Check sheet for the modelled part. Datum: model origin and axes. Units: mm. A direction names the side the tool comes from. Round coordinates to 2 decimals unless told otherwise and drop trailing zeros. Loops run counter-clockwise (first coordinate to the right, second up) from the corner with the lowest first, then second, coordinate; pieces in that order, holes last. Notation, with made-up numbers: (87.25, 67.5) - (107.25, 67.5) arc R19 cw to (107.25, 98.5) - close; hole circle Ø3 at (62.5, 38.25). An arc over 180 degrees is marked (long way). Answer in a Markdown table with one row per item. Add a question column.
(1) Access from +Z, -Z, +X, -X, +Y, -Y to the whole of each face (thin tool, end or side, straight path). Record for faces 5 (the flat face through (-39, 18, -33.975)), 6 (the flat face through (-39, 5.2, -51)), 7 (the flat face through (-39, 3, -56)).
(2) Cross-section at D-D on y = 11.5. Enter the section's corners in (x, z), then the cut area to 3 significant figures.
(3) Cross-section at B-B on z = -6. Enter the section's corners in (x, y).
(4) Cross-section at A-A on x = -43. Enter the section's corners in (y, z), then the cut area to 3 significant figures.
(5) Cross-section at C-C on x = -37.25. Enter the section's corners in (y, z).
(6) Gauge pin test, flat ends, axial feed: pin 1 (5 mm diameter, centred on x = -43, z = -50, fed in from +Y); pin 2 (12 mm diameter, centred on x = -33.5, z = -19.5, fed in from +Y); pin 3 (3 mm diameter, centred on x = -45, y = 19.5, fed in from +Z). Record the tip position at first contact, or that the pin passes through.
(7) Mould release check, pull along X, two halves, no side actions. Record for faces 1 (the cylindrical face through (-42.26, 2.64, -48.58)), 2 (the flat face through (-39, 21.2, -35)), 3 (the cylindrical face through (-43.35, 2.64, -4.44)), 4 (the cylindrical face through (-26.57, 2.64, -55.4)): +X half, -X half, draft (parallel to the pull), parting line (faces both ways), or undercut.
(8) Thickness scan on line 1 along Z through (x, y) = (-43, 3.05); line 2 along X through (y, z) = (1.5, -6); line 3 along Y through (x, z) = (-47, -17.5). Record the ranges inside material, lowest first.
Autodesk Inventor part; units mm, degrees
ref_plane "YZ Plane" through (0, 0, 0) normal (1, 0, 0) x (0, 1, 0)
ref_plane "XZ Plane" through (0, 0, 0) normal (0, 1, 0) x (-1, 0, 0)
ref_plane "XY Plane" through (0, 0, 0) normal (0, 0, 1) x (1, 0, 0)
sketch "Эскиз1" plane through (0, 0, 0) normal (0, 1, 0) x (-1, 0, 0)
  line L0 (0, 0) -> (52, 0)
  line L1 (52, 0) -> (52, -56)
  line L2 (52, -56) -> (0, -56)
  line L3 (0, -56) -> (0, 0)
  dimension "d0" = 56
  dimension "d9" = 52
extrude "Выдавливание1" add sketch "Эскиз1" along normal blind 5.2
ref_plane "РабПлоскость2" through (0, 3.2, -12) normal (0, -1, 0) x (1, 0, 0)
fillet "Сопряжение1" radius 2 4 edges at (0, 2.6, 0) (0, 2.6, -56) (-52, 2.6, -56) (-52, 2.6, 0)
ref_plane "РабПлоскость1" through (0, 0, -12) normal (1, 0, 0) x (0, 0, -1)
sketch "Эскиз4" plane through (0, 0, -12) normal (1, 0, 0) x (0, 0, -1)
  line L0 (34.9749, 5.2) -> (21.9749, 5.2)
  line L1 (21.9749, 21.2) -> (21.9749, 5.2)
  arc A0 (24.5222, 21.2) -> (34.9749, 5.2) centre (138.2876, 84.1082) ccw
  line L2 (21.9749, 21.2) -> (24.5222, 21.2)
  line L3 (44, 0) -> (44, 5.2)
  point P0 (-12, 0)
  dimension "d26" = 13
  dimension "d35" = 130
  dimension "d43" = 9.0251
extrude "Выдавливание4" add sketch "Эскиз4" against normal up to surface (52 mm away)
sketch "Эскиз5" plane through (0, 0, 0) normal (0, -1, 0) x (1, 0, 0)
  line L0 (0, 0) -> (-26, 0)
  line L1 (-26, 0) -> (-26, -56)
  line L2 (-26, -56) -> (0, -56)
  line L3 (0, -56) -> (0, 0)
  dimension "d37" = 26
extrude "Выдавливание5" cut sketch "Эскиз5" against normal blind 34
fillet "Сопряжение4" radius 2 2 edges at (-26, 2.6, 0) (-26, 2.6, -56)
fillet "Сопряжение5" radius 10 1 edges at (-39, 5.2, -33.9749)
sketch "Эскиз6" plane through (0, 5.2, 0) normal (0, 1, 0) x (1, 0, 0)
  circle A0 centre (-43, 6) radius 1.6
  circle A1 centre (-43, 50) radius 1.6
  line L0 (-52, 54) -> (-52, 46.9749)
  line L1 (-52, 23.9749) -> (-52, 2)
  line L2 (-50, 0) -> (-28, 0)
  line L3 (-28, 56) -> (-50, 56)
  point P0 (0, 0)
  dimension "d45" = 3.2
  dimension "d46" = 3.2
  dimension "d47" = 9
  dimension "d48" = 9
  dimension "d49" = 6
  dimension "d50" = 6
extrude "Выдавливание6" cut sketch "Эскиз6" against normal blind 40
properties part number "порожек"
Answers:
| question | item | result |
|---|---|---|
| 1 | face 5 | +Z, +X, -X, +Y |
| 1 | face 6 | -Z, +X, -X, +Y |
| 1 | face 7 | -Z, +X, -X, +Y, -Y |
| 2 | outline | (-52, -42.45) - (-26, -42.45) - (-26, -33.27) - (-52, -33.27) - close |
| 2 | area | 239 mm^2 |
| 3 | outline | (-52, 0) - (-44.6, 0) - (-44.6, 5.2) - (-52, 5.2) - close; (-41.4, 0) - (-26, 0) - (-26, 5.2) - (-41.4, 5.2) - close |
| 4 | outline | (0, -56) - (5.2, -56) - (5.2, -51.6) - (0, -51.6) - close; (0, -48.4) - (5.2, -48.4) - (5.2, -46.97) arc R130.01 cw to (21.2, -36.52) - (21.2, -33.97) - (15.2, -33.97) arc R10 cw to (5.2, -23.97) - (5.2, -7.6) - (0, -7.6) - close; (0, -4.4) - (5.2, -4.4) - (5.2, 0) - (0, 0) - close |
| 4 | area | 399 mm^2 |
| 5 | outline | (0, -56) - (5.2, -56) - (5.2, -46.97) arc R130.01 cw to (21.2, -36.52) - (21.2, -33.97) - (15.2, -33.97) arc R10 cw to (5.2, -23.97) - (5.2, 0) - (0, 0) - close |
| 6 | pin 1 | stops at y = 5.2 |
| 6 | pin 2 | stops at y = 5.32 |
| 6 | pin 3 | stops at z = -33.97 |
| 7 | face 1 | undercut |
| 7 | face 2 | draft |
| 7 | face 3 | undercut |
| 7 | face 4 | +X half |
| 8 | line 1 | z = -56 to -51.6, -48.4 to -7.6, -4.4 to 0 |
| 8 | line 2 | x = -52 to -44.6, -41.4 to -26 |
| 8 | line 3 | y = 0 to 5.2 |
